Work out the finished part from the listing and answer in its coordinate system (mm). A direction names the side the tool comes from. Coordinates: 2 decimals unless noted, no trailing zeros. Order: outer loops, then holes, each group sorted by start corner. A loop starts at its lowest first (then second) coordinate and runs counter-clockwise, first axis right, second up. Notation, with made-up numbers: (79.5, -32.75) - (108.5, -32.75) arc R24 ccw to (108.5, -20.75) - close; hole circle Ø7 at (13.25, 80.5). An arc over 180 degrees is marked (long way). Answer as a JSON object with one key per item and string values. Group by question number.
1) A tool of negligible diameter and unlimited length cuts with its end or side. For faces 5 (the face through (15, -10.339, 17)), 6 (the face through (22, -18, 28.524)), 7 (the face through (15, -18, 0)), 8 (the face through (16, -5.241, 14)), 9 (the face through (25.353, -18, 14)), from which of +Z, -Z, +X, -X, +Y, -Y can it reach the whole face along a straight path? Write none if from no direction.
2) Section A-A (z = 15) is taken. Give the vertices of the cut face in (x, y).
3) Each of these flat-tipped pins is pushed along its axis until it touches: P1, Ø1.5, axis at x = 11.5, z = 9, coming from the -Y side; P2, Ø4.5, axis at x = 15.5, y = -18, coming from the +Z side; P3, Ø5, axis at y = -30, z = 13, coming from the +X side. Where does it stop, or does it pass through?
4) Section B-B (y = -32.5) is taken. Give the vertices of the cut face in (x, z), plus the area to 3 significant figures.
5) Section D-D (x = 14.5) is taken. Give the vertices of the cut face in (y, z).
6) The mould has two halves that part along X. Classify faces 1 (the face through (19.971, -18, 17)), 2 (the face through (5.807, -18, 14)), 3 (the face through (30.735, -18, 3)), 4 (the face through (15, -35.834, 26)): released by +X, released by -X, zero draft, split by the parting line, or undercut.
7) Section C-C (x = 4.5) is taken. Give the vertices of the cut face in (y, z), plus the area to 3 significant figures.
8) Find the intervals of material crossed by line 1 along Z through (x, y) = (13.5, -2); line 2 along X through (y, z) = (-19, 20.5); line 3 along Y through (x, z) = (18, 14.25), in increasing order.
from build123d import *

# Parameters (mm, degrees)
F0_W     = 30.7351611555
F0_H     = 5.5238311179
F1_DEPTH = 36
F3_DEPTH = 18
F4_W     = 30.7351611555
F4_H     = 35.8340851963
F4_W_2   = 9.0647470206
F4_H_2   = 15.0134908035
F5_DEPTH = 5


with BuildPart() as f1:
    # F0 (on Front) → F1 (new body)
    with BuildSketch(Plane.XZ):
        with Locations((15.3675805777, 2.7619155589)):
            Rectangle(F0_W, F0_H)
    extrude(amount=F1_DEPTH)

    # F2 (on face) → F3 (join)
    with BuildSketch(Plane.XY.offset(5.5238311179)):
        Polygon((25.3529716283, -30.4518900812), (25.3529716283, -18), (25.3529716283, -5.2405577153), (5.8071063831, -5.2405577153), (5.8071063831, -30.4518900812), align=None)
        Polygon((19.9707727879, -25.3529697657), (15.5800390057, -25.3529697657), (10.9060257673, -25.3529697657), (10.9060257673, -10.3394789621), (19.9707727879, -10.3394789621), align=None, mode=Mode.SUBTRACT)
    extrude(amount=F3_DEPTH)

    # F4 (on face) → F5 (join)
    with BuildSketch(Plane.XY.offset(23.5238311179)):
        with Locations((15.3675805777, -17.9170425981)):
            Rectangle(F4_W, F4_H)
        with Locations((15.4383992776, -17.8462243639)):
            Rectangle(F4_W_2, F4_H_2, mode=Mode.SUBTRACT)
    extrude(amount=F5_DEPTH)


solid = f1.part
Report:
{
 "1": {"face 5": "+Z", "face 6": "+Z, +X, -X, +Y, -Y", "face 7": "-Z, +X, -X, +Y, -Y", "face 8": "+X, -X, +Y", "face 9": "+X, +Y, -Y"},
 "2": {"outline": "(5.81, -30.45) - (25.35, -30.45) - (25.35, -5.24) - (5.81, -5.24) - close; hole (10.91, -25.35) - (19.97, -25.35) - (19.97, -10.34) - (10.91, -10.34) - close"},
 "3": {"P1": "stops at y = -30.45", "P2": "stops at z = 5.52", "P3": "stops at x = 25.35"},
 "4": {"outline": "(0, 0) - (30.74, 0) - (30.74, 5.52) - (0, 5.52) - close; (0, 23.52) - (30.74, 23.52) - (30.74, 28.52) - (0, 28.52) - close", "area": "323 mm²"},
 "5": {"outline": "(-36, 0) - (0, 0) - (0, 5.52) - (-5.24, 5.52) - (-5.24, 23.52) - (0, 23.52) - (0, 28.52) - (-10.34, 28.52) - (-10.34, 5.52) - (-25.35, 5.52) - (-25.35, 28.52) - (-35.83, 28.52) - (-35.83, 23.52) - (-30.45, 23.52) - (-30.45, 5.52) - (-36, 5.52) - close"},
 "6": {"face 1": "undercut", "face 2": "released by -X", "face 3": "released by +X", "face 4": "zero draft"},
 "7": {"outline": "(-36, 0) - (0, 0) - (0, 5.52) - (-36, 5.52) - close; (-35.83, 23.52) - (0, 23.52) - (0, 28.52) - (-35.83, 28.52) - close", "area": "378 mm²"},
 "8": {"line 1": "z = 0 to 5.52, 23.52 to 28.52", "line 2": "x = 5.81 to 10.91, 19.97 to 25.35", "line 3": "y = -30.45 to -25.35, -10.34 to -5.24"}
}
